Drawing for the job (mm, zero at the part's lowest x, y, z). Give positions to 0.01 mm unless a question says otherwise; leave off trailing zeros. Write each loop counter-clockwise with the first axis right and the second up, starting at its lowest first coordinate (ties: lowest second). Pieces come first, ordered by that corner, then holes. Notation, with made-up numbers: (54, 9.25) - (61, 9.25) arc R20 ccw to (61, 46.25) - close; hole circle Ø2 at (88.25, 15). An arc over 180 degrees is marked (long way). Answer as a JSON object with one key per item and string values. Group by question number.
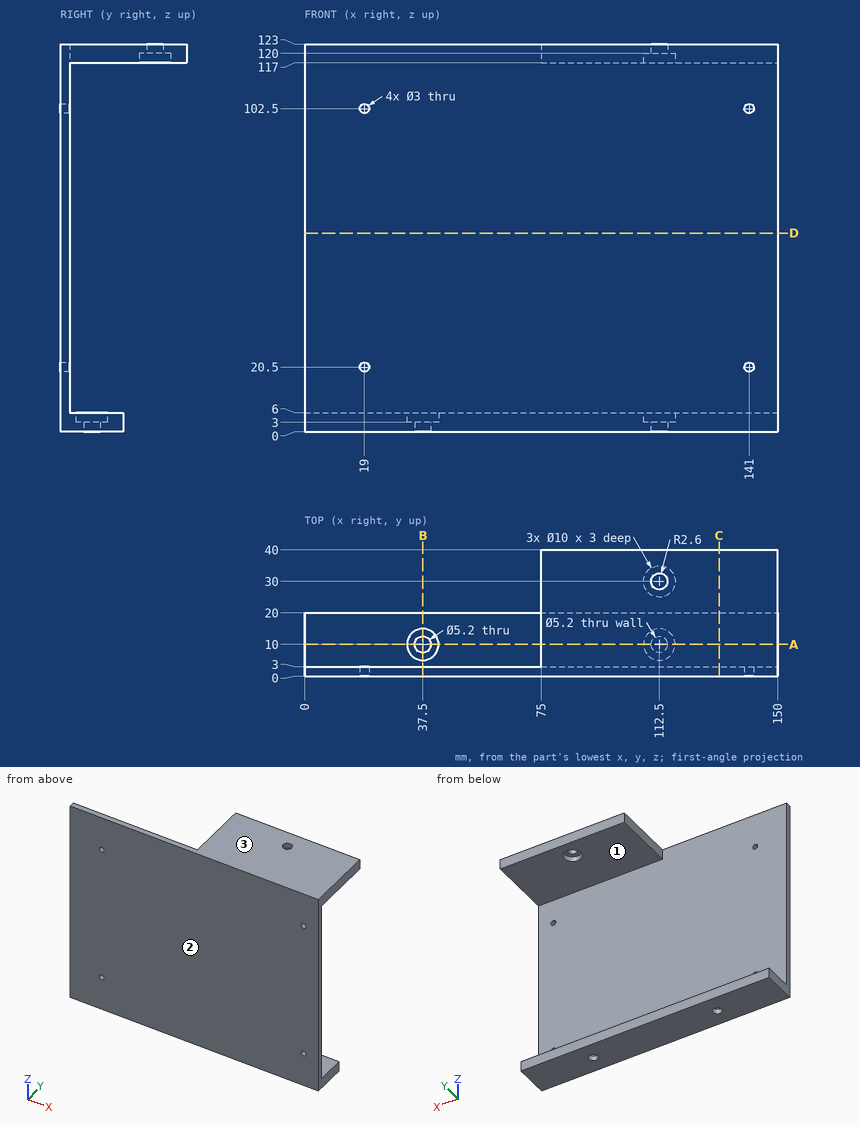
1) Probe line 1 (X direction, y = 1.45, z = 20.5); line 2 (Z direction, x = 141, y = 1.15); line 3 (Z direction, x = 95.5, y = 13). List the from-to ranges inside material, lowest first.
2) Drop flat-ended pins along their axis: P1, Ø3, axis at x = 113.5, y = 32, coming from the -Z side; P2, Ø8, axis at x = 36.5, y = 7.5, coming from the +Z side; P3, Ø5, axis at x = 19, z = 102.5, coming from the +Y side; P4, Ø13, axis at x = 37.5, y = 10, coming from the -Z side. Give the stop position or say it passes through.
3) Mould opens along Z. For the marked faces 1, 2 and 3 say: pulls with the +Z half, pulls with the -Z half, needs draft (parallel to the pull), parting line crosses it, or undercut.
4) Band-saw the part on A-A (y = 10). List the corners of the cut face in (x, z).
5) Band-saw the part on B-B (x = 37.5). List the corners of the cut face in (y, z), plus the area to 3 significant figures.
6) Band-saw the part on C-C (x = 131.5). List the corners of the cut face in (y, z).
7) Band-saw the part on D-D (z = 63). List the corners of the cut face in (x, y).
Verdict:
{
 "1": {"line 1": "0 to 17.5, 20.5 to 139.5, 142.5 to 150", "line 2": "0 to 19, 22 to 101, 104 to 123", "line 3": "0 to 6, 117 to 123"},
 "2": {"P1": "z = 120", "P2": "z = 6", "P3": "y = 3", "P4": "z = 0"},
 "3": {"face 1": "undercut", "face 2": "needs draft", "face 3": "pulls with the +Z half"},
 "4": {"outline": "(0, 0) - (34.9, 0) - (34.9, 3) - (32.5, 3) - (32.5, 6) - (0, 6) - close; (40.1, 0) - (109.9, 0) - (109.9, 3) - (107.5, 3) - (107.5, 6) - (42.5, 6) - (42.5, 3) - (40.1, 3) - close; (75, 117) - (150, 117) - (150, 123) - (75, 123) - close; (115.1, 0) - (150, 0) - (150, 6) - (117.5, 6) - (117.5, 3) - (115.1, 3) - close"},
 "5": {"outline": "(0, 0) - (7.4, 0) - (7.4, 3) - (5, 3) - (5, 6) - (3, 6) - (3, 123) - (0, 123) - close; (12.6, 0) - (20, 0) - (20, 6) - (15, 6) - (15, 3) - (12.6, 3) - close", "area": "425 mm2"},
 "6": {"outline": "(0, 0) - (20, 0) - (20, 6) - (3, 6) - (3, 117) - (40, 117) - (40, 123) - (0, 123) - close"},
 "7": {"outline": "(0, 0) - (150, 0) - (150, 3) - (0, 3) - close"}
}
